For this review, use the dimensioned drawing (mm, ordinates from the lowest corner) and the shaded views. Round coordinates to 2 decimals unless told otherwise and drop trailing zeros. Loops run counter-clockwise (first coordinate to the right, second up) from the corner with the lowest first, then second, coordinate; pieces in that order, holes last. Notation, with made-up numbers: (7, 62) - (34, 62) arc R10 cw to (34, 71) - close; hole circle Ø4 at (45, 68.5). An arc over 180 degrees is marked (long way). Use one line per item in the form item = value. Start each with the question number.
(1) The part is to be moulded in two halves that separate along Z. For the marked faces 1 and 2, say which applies: released by +Z, released by -Z, zero draft, split by the parting line, or undercut.
(2) Wall thickness on probe 1 along Y at (x, z) = (3, 1.15); probe 2 along X at (y, z) = (40, 0.45); probe 3 along X at (y, z) = (14.5, 0.5): over which ranges is each line inside the solid? List them lowest first. Write a range as [from, to].
(3) We need section A-A, the plane y = 27. Write out the cut boundary in (x, z).
(4) We need section D-D, the plane y = 34. Write out the cut boundary in (x, z), then the cut area to 3 significant figures.
(5) We need section B-B, the plane x = 29. Write out the cut boundary in (y, z), then the cut area to 4 significant figures.
(6) We need section C-C, the plane y = 14. Write out the cut boundary in (x, z).
(7) For pin 1 (0.9 mm diameter, centred on y = 6, z = 1, fed in from +X), flat-tipped, find the tip position at first contact; note if it passes through.
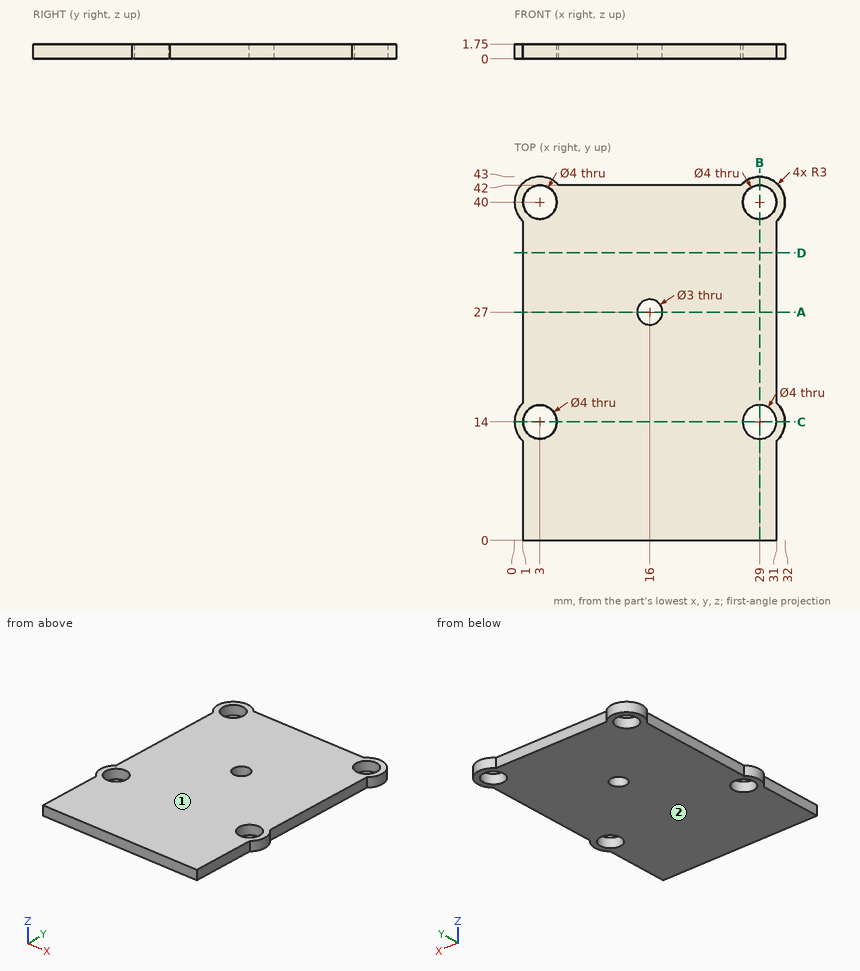
Data:
q1.face_1 = released by +Z
q1.face_2 = released by -Z
q2.probe_1 = [0, 12], [16, 38], [42, 43]
q2.probe_2 = [0, 1], [5, 27], [31, 32]
q2.probe_3 = [0.04, 1.06], [4.94, 27.06], [30.94, 31.96]
q3.outline = (1, 0) - (14.5, 0) - (14.5, 1.75) - (1, 1.75) - close; (17.5, 0) - (31, 0) - (31, 1.75) - (17.5, 1.75) - close
q4.outline = (1, 0) - (31, 0) - (31, 1.75) - (1, 1.75) - close
q4.area = 52.5 mm^2
q5.outline = (0, 0) - (12, 0) - (12, 1.75) - (0, 1.75) - close; (16, 0) - (38, 0) - (38, 1.75) - (16, 1.75) - close; (42, 0) - (43, 0) - (43, 1.75) - (42, 1.75) - close
q5.area = 61.25 mm^2
q6.outline = (0, 0) - (1, 0) - (1, 1.75) - (0, 1.75) - close; (5, 0) - (27, 0) - (27, 1.75) - (5, 1.75) - close; (31, 0) - (32, 0) - (32, 1.75) - (31, 1.75) - close
q7.pin_1 = 31
